Build history of the part. All positions in model axes, mm. A direction names the side the tool comes from. Give positions to 0.01 mm unless a question says otherwise; leave off trailing zeros. Write each loop counter-clockwise with the first axis right and the second up, starting at its lowest first coordinate (ties: lowest second). Pieces come first, ordered by that corner, then holes.
from build123d import *

# Parameters (mm, degrees)
F0_R        = 2.15
F1_DEPTH    = 10
F2_W        = 3.75
F2_H        = 5.8
F3_DEPTH    = 5
F4_R        = 1.45
F5_DEPTH    = 25
F6_T1_DEPTH = 20


# Not quite as in the source:
# - a fillet or chamfer that OpenCascade refuses, or shapes differently, is made with other operations: its cross-section is extruded or revolved along the edge and cut away or added


with BuildPart() as f1:
    # F0 (on Top) → F1 (new body)
    with BuildSketch(Plane.XY):
        with BuildLine():
            Line((-7.6355537636, 34.15), (-7.6355537636, 0))
            Line((-7.6355537636, 0), (1.8644462364, 0))
            Line((1.8644462364, 0), (1.8644462364, 2.2661458509))
            ThreePointArc((1.8644462364, 2.2661458509), (-2.9359075253, 15.6540914389), (10.1144462364, 10))
            ThreePointArc((10.1144462364, 10), (8.0185376754, 4.6996462382), (2.8644462364, 2.2661458509))
            Line((2.8644462364, 2.2661458509), (2.8644462364, 0))
            Line((2.8644462364, 0), (12.3644462364, 0))
            Line((12.3644462364, 0), (12.3644462364, 34.15))
            Line((12.3644462364, 34.15), (-7.6355537636, 34.15))
        make_face()
        with Locations((2.3644462364, 24.15)):
            Circle(F0_R, mode=Mode.SUBTRACT)
        with BuildLine():
            ThreePointArc((10.1144462364, 10), (-2.9359075253, 15.6540914389), (1.8644462364, 2.2661458509))
            Line((1.8644462364, 2.2661458509), (1.8644462364, 5.880230589))
            ThreePointArc((1.8644462364, 5.880230589), (-0.387598458, 13.1062437123), (6.5144462364, 10))
            ThreePointArc((6.5144462364, 10), (5.4706899487, 7.2479553056), (2.8644462364, 5.880230589))
            Line((2.8644462364, 5.880230589), (2.8644462364, 2.2661458509))
            ThreePointArc((2.8644462364, 2.2661458509), (8.0185376754, 4.6996462382), (10.1144462364, 10))
        make_face()
    extrude(amount=F1_DEPTH)

    # F2 (on face) → F3 (join)
    with BuildSketch(Plane.XY.offset(10)):
        with Locations((-5.7605537636, 24.15)):
            Rectangle(F2_W, F2_H)
        with Locations((10.4894462364, 24.15)):
            Rectangle(F2_W, F2_H)
    extrude(amount=F3_DEPTH)

    # F4 (on face) → F5 (cut)
    with BuildSketch(Plane.YZ.offset(12.3644462364)):
        with Locations((2.95, 5)):
            Circle(F4_R)
    extrude(amount=-F5_DEPTH, mode=Mode.SUBTRACT)

    # F6: fillet of radius 2 on 4 edges, made by hand

    # F6_s2 → F6_t1 (cut)
    with BuildSketch(Plane.XY.offset(-5)):
        with BuildLine():
            ThreePointArc((12.3644462364, 2), (11.7786597988, 0.5857864376), (10.3644462364, 0))
            Line((10.3644462364, 0), (12.3644462364, 0))
            Line((12.3644462364, 0), (12.3644462364, 2))
        make_face()
        with BuildLine():
            ThreePointArc((-7.6355537636, 2), (-7.0497673259, 0.5857864376), (-5.6355537636, 0))
            Line((-5.6355537636, 0), (-7.6355537636, 0))
            Line((-7.6355537636, 0), (-7.6355537636, 2))
        make_face()
        with BuildLine():
            ThreePointArc((10.3644462364, 34.15), (11.7786597988, 33.5642135624), (12.3644462364, 32.15))
            Line((12.3644462364, 32.15), (12.3644462364, 34.15))
            Line((12.3644462364, 34.15), (10.3644462364, 34.15))
        make_face()
        with BuildLine():
            ThreePointArc((-5.6355537636, 34.15), (-7.0497673259, 33.5642135624), (-7.6355537636, 32.15))
            Line((-7.6355537636, 32.15), (-7.6355537636, 34.15))
            Line((-7.6355537636, 34.15), (-5.6355537636, 34.15))
        make_face()
    extrude(amount=F6_T1_DEPTH, mode=Mode.SUBTRACT)


solid = f1.part
(1) Saw through at A-A, the plane y = 2.95. List the corners of the cut face in (x, z).
(2) Drop flat-ended pins along their axis: pin 1 (3 mm diameter, centred on x = 10, z = 12, fed in from +Y); pin 2 (2.5 mm diameter, centred on y = 2.95, z = 5, fed in from +X); pin 3 (1.9 mm diameter, centred on x = 10.5, z = 12, fed in from -Y); pin 4 (1 mm diameter, centred on x = -2.5, y = 9, fed in from +Z). Give the stop position or say it passes through.
(3) Saw through at B-B, the plane z = 11. List the corners of the cut face in (x, y).
(4) 3-axis set-ups, long thin cutter, end or side, ignore diameter. For faces 5 (the face through (8.614, 24, 12)), 6 (the face through (-6, 21.25, 12)), 7 (the face through (2.864, 4.3, 3.8)): which of +Z, -Z, +X, -X, +Y, -Y reach the whole face in a straight line?
(5) Probe line 1 (Y direction, x = 7, z = 5); line 2 (Y direction, x = 1, z = 8.5); line 3 (X direction, y = 26.5, z = 12). List the from-to ranges inside material, lowest first.
(6) Saw through at D-D, the plane z = 5. List the corners of the cut face in (x, y).
(7) Saw through at C-C, the plane y = 24.15. List the corners of the cut face in (x, z), plus the area to 4 significant figures.
(8) Mould opens along Y. For faces 1 (the face through (-6, 27.05, 12)), 2 (the face through (-2, 0, 5)), 3 (the face through (-3.886, 24, 12)), 4 (the face through (1.9, 22.05, 4.93)) say: +Y half, -Y half, draft (parallel to the pull), parting line (faces both ways), or undercut.
Computed values:
1. outline: (-7.64, 0) - (1.86, 0) - (1.86, 3.55) - (-7.64, 3.55) - close; (-7.64, 6.45) - (1.86, 6.45) - (1.86, 10) - (-7.64, 10) - close; (2.86, 0) - (12.36, 0) - (12.36, 3.55) - (2.86, 3.55) - close; (2.86, 6.45) - (12.36, 6.45) - (12.36, 10) - (2.86, 10) - close
2. pin 1: stops at y = 27.05
2. pin 2: passes through
2. pin 3: stops at y = 21.25
2. pin 4: stops at z = 10
3. outline: (-7.64, 21.25) - (-3.89, 21.25) - (-3.89, 27.05) - (-7.64, 27.05) - close; (8.61, 21.25) - (12.36, 21.25) - (12.36, 27.05) - (8.61, 27.05) - close
4. face 5: +Z, +Y, -Y
4. face 6: +Z, +X, -X, -Y
4. face 7: +Z, -Z, -Y
5. line 1: y = 0 to 1.5, 4.4 to 34.15
5. line 2: y = 0 to 6.08, 13.92 to 22.49, 25.81 to 34.15
5. line 3: x = -7.64 to -3.89, 8.61 to 12.36
6. outline: (-7.64, 4.4) - (1.86, 4.4) - (1.86, 5.88) arc R4.15 cw (long way) to (2.86, 5.88) - (2.86, 4.4) - (12.36, 4.4) - (12.36, 32.15) arc R2 ccw to (10.36, 34.15) - (-5.64, 34.15) arc R2 ccw to (-7.64, 32.15) - close; (-7.57, 1.5) arc R2 ccw to (-5.64, 0) - (1.86, 0) - (1.86, 1.5) - close; (2.86, 0) - (10.36, 0) arc R2 ccw to (12.3, 1.5) - (2.86, 1.5) - close; hole circle Ø4.3 at (2.36, 24.15)
7. outline: (-7.64, 0) - (0.21, 0) - (0.21, 10) - (-3.89, 10) - (-3.89, 15) - (-7.64, 15) - close; (4.51, 0) - (12.36, 0) - (12.36, 15) - (8.61, 15) - (8.61, 10) - (4.51, 10) - close
7. area: 194.5 mm2
8. face 1: +Y half
8. face 2: -Y half
8. face 3: draft
8. face 4: undercut
